Can you work these out from the model? Positions are in its coordinate system, mm. A direction names the side the tool comes from. Coordinates: 2 decimals unless noted, no trailing zeros. Loops run counter-clockwise (first coordinate to the right, second up) from the corner with the lowest first, then second, coordinate; pieces in that order, holes last. Notation, with made-up numbers: M -12,9.25 L 9,9.25 A30 cw 9,48.25 Z; hole C -30,76 d2. An arc over 180 degrees is marked long. Answer as a JSON object with one key per item and string values. Group by question number.
Item 1: Suppose I cut it at A-A (y = 8.75). Write out the boundary of the cut face in (x, z).
Item 2: Suppose I cut it at B-B (x = 5). Write out the boundary of the cut face in (y, z), then the cut area to 3 significant figures.
Item 3: Suppose I cut it at D-D (x = 1.5). Write out the boundary of the cut face in (y, z).
Item 4: Which directions (+Z, -Z, +X, -X, +Y, -Y) give clear straight access to the entire face, cutting with the end or side of a thin tool? Please do faces 1 (the flat face through (5, 10, -18)), 2 (the flat face through (0, 6, -20)).
Item 5: I'm going to push flat-ended pins straight in: pin 1 Ø5.5 at (x, z) = (5, -18) entering from -Y; pin 2 Ø4 at (x, z) = (6.5, -13.5) entering from -Y; pin 3 Ø4 at (x, z) = (3.5, -13.5) entering from +Y. Where does each tip first touch, or does it pass through?
Item 6: We'd pull the mould along Z, two halves only. Please class faces 3 (the flat face through (5, 0, -22)), 4 (the flat face through (5, 8, -30)), 5 (the cylindrical face through (4.35, 4.93, -20.93)), 6 (the flat face through (5, 6, -10)): +Z half, -Z half, draft (parallel to the pull), parting line (faces both ways), or undercut.
Item 7: Suppose I cut it at C-C (z = -18). Write out the boundary of the cut face in (x, y).
Item 8: If I drill on line 1 (Z direction, x = 5, y = 4.5); line 2 (Z direction, x = 3, y = 3.75); line 3 (X direction, y = 5, z = -20.75), over which ranges is the centre line in solid material (lowest first)?
```python
from build123d import *

# Parameters (mm, degrees)
EXTRUDE_1_DEPTH     = 10
EXTRUDE_2_DEPTH     = 10
SKETCH_2_R          = 3
CUT_EXTRUDE_1_DEPTH = 10


with BuildPart() as part:
    # 草图1 → 凸台-拉伸1 (new body)
    with BuildSketch(Plane(origin=(0, 0, 0), x_dir=(0, 0, -1), z_dir=(1, 0, 0))):
        with BuildLine():
            Line((10, 12), (10, 0))
            Line((10, 0), (30, 0))
            Line((30, 0), (30, 15.532515952))
            ThreePointArc((30, 15.532515952), (20.077840204, 13.3255511), (10, 12))
        make_face()
    extrude(amount=EXTRUDE_1_DEPTH)

    # 草图1<2> → 凸台-拉伸2 (add)
    with BuildSketch(Plane(origin=(0, 0, 0), x_dir=(0, 0, -1), z_dir=(1, 0, 0))):
        with BuildLine():
            Line((10, 12), (10, 0))
            Line((10, 0), (30, 0))
            Line((30, 0), (30, 15.532515952))
            ThreePointArc((30, 15.532515952), (20.077840204, 13.3255511), (10, 12))
        make_face()
    extrude(amount=EXTRUDE_2_DEPTH)

    # 草图2 → 切除-拉伸1 (cut)
    with BuildSketch(Plane.XZ):
        with Locations((5, -18)):
            Circle(SKETCH_2_R)
    extrude(amount=-CUT_EXTRUDE_1_DEPTH, mode=Mode.SUBTRACT)


solid = part.part
```
From the geometry:
{
 "1": {"outline": "M 0,-30 L 10,-30 L 10,-10 L 0,-10 Z; hole C 5,-18 d6"},
 "2": {"outline": "M 0,-30 L 15.53,-30 A115.43 cw 12,-10 L 0,-10 L 0,-15 L 10,-15 L 10,-21 L 0,-21 Z", "area": "209 mm2"},
 "3": {"outline": "M 0,-30 L 15.53,-30 A115.43 cw 12,-10 L 0,-10 Z"},
 "4": {"face 1": "-Y", "face 2": "+Z, -Z, -X, +Y, -Y"},
 "5": {"pin 1": "y = 10", "pin 2": "y = 0", "pin 3": "y = 12.61"},
 "6": {"face 3": "draft", "face 4": "-Z half", "face 5": "undercut", "face 6": "+Z half"},
 "7": {"outline": "M 0,0 L 2,0 L 2,10 L 8,10 L 8,0 L 10,0 L 10,12.98 L 0,12.98 Z"},
 "8": {"line 1": "-30 to -21, -15 to -10", "line 2": "-30 to -20.24, -15.76 to -10", "line 3": "0 to 3.8, 6.2 to 10"}
}
